Check sheet for the modelled part. Datum: model origin and axes. Units: mm. A direction names the side the tool comes from. Give positions to 0.01 mm unless a question says otherwise; leave off trailing zeros. Write each loop counter-clockwise with the first axis right and the second up, starting at its lowest first coordinate (ties: lowest second). Pieces come first, ordered by that corner, then holes. Notation, with made-up numbers: M 7.25,48.25 L 30.25,48.25 A32 cw 30.25,75.25 Z; hole C 21.5,-26.75 d4. An arc over 180 degrees is marked long. Write item = value, one per line. Start each with the question number.
1) Sectioned sample at D-D, the plane z = 8.25. Record the cut outline in (x, y) (1 decimal).
2) Scan lines: L1, parallel to Y at x = 0, z = 0.25; L2, parallel to Z at x = -18, y = -21; L3, parallel to Z at x = 15.5, y = -6.5. Record each from-to range of solid material in increasing order.
3) Sectioned sample at A-A, the plane x = 0. Record the cut outline in (y, z), then the cut area to 3 significant figures.
4) Set-up check for faces 4 (the face through (-29.97, 1.32, -0.03)), 5 (the face through (-1.12, -5.043, 6.553)): record each of +Z, -Z, +X, -X, +Y, -Y from which the full face is reachable in a straight line by a thin tool's end or side.
5) Sectioned sample at C-C, the plane z = 4.5. Record the cut outline in (x, y) (3 decimals).
6) Gauge pin test, flat ends, axial feed: pin 1 (2 mm diameter, centred on x = 21.5, z = -2.5, fed in from -Y); pin 2 (3 mm diameter, centred on x = 0, y = 0, fed in from -Z); pin 3 (5 mm diameter, centred on x = -4.5, z = 0.5, fed in from -Y); pin 4 (4 mm diameter, centred on x = -23.5, y = -0.5, fed in from -Z). Record the tip position at first contact, or that the pin passes through.
7) Draft check along Z on faces 1 (the face through (0, 2, 0)), 2 (the face through (25.865, -10.724, -0.006)), 3 (the face through (-0.7, -3.3, -9.1)). Enter one of: pulls with the +Z half, pulls with the -Z half, needs draft (parallel to the pull), parting line crosses it, or undercut.
from build123d import *

# Parameters (mm, degrees)
F3_D = 4
F4_T = -2


with BuildPart() as f1:
    # F0 (on Front) → F1 (revolve)
    with BuildSketch(Plane.XZ):
        Polygon((0, 10), (0, 0), (30, 0), (30, 2), align=None)
    revolve(axis=Axis((0, 0, 5), (0, 0, 1)))

    # F3 (through all)
    with Locations(Plane(origin=(0, 0, 0), x_dir=(1, 0, 0), z_dir=(0, 0, -1))):
        with Locations((0, 0)):
            Hole(F3_D / 2)

    # F4
    f4_openings = [f1.faces().sort_by_distance(p)[0] for p in [
        (-29.151472, 0, 0),
    ]]
    offset(amount=F4_T, openings=f4_openings)

    # F5: F1 across plane


with BuildPart() as f1_1:
    add(f1.part)
    add(f1.part.mirror(Plane.XY))


solid = f1_1.part
Data:
q1.outline = C 0,0 d13.1; hole C 0,0 d4
q2.L1 = -30 to -28, -4 to -2, 2 to 4, 28 to 30
q2.L2 = -2.62 to -0.55, 0.55 to 2.62
q2.L3 = -5.52 to -3.45, 3.45 to 5.52
q3.outline = M -30,-2 L -2,-9.47 L -2,9.47 L -30,2 Z; M 2,-9.47 L 30,-2 L 30,2 L 2,9.47 Z; hole M -28,-0.46 L -4,-6.86 L -4,6.86 L -28,0.46 Z; hole M 4,-6.86 L 28,-0.46 L 28,0.46 L 4,6.86 Z
q3.area = 290 mm2
q4.face_4 = +Z, -Z
q4.face_5 = none
q5.outline = C 0,0 d41.25; C 0,0 d8; hole C 0,0 d25.726; hole C 0,0 d4
q6.pin_1 = -21.78
q6.pin_2 = through
q6.pin_3 = -29.93
q6.pin_4 = -4.27
q7.face_1 = needs draft
q7.face_2 = undercut
q7.face_3 = pulls with the -Z half
